Can you work these out from the model? Positions are in its coordinate system, mm. Face numbers are marked on the shaded views. A direction names the side the tool comes from. Coordinates: 2 decimals unless noted, no trailing zeros. Order: outer loops, then holes, each group sorted by start corner. A loop starts at its lowest first (then second) coordinate and runs counter-clockwise, first axis right, second up. Notation, with made-up numbers: M -23.75,89.25 L 1.25,89.25 A28 ccw 1.25,124.25 Z; hole C 47.25,-7.5 d4. An arc over 180 degrees is marked long. Answer as CSV lines item,"result". Start each with the question number.
1. If we section it at A-A (y = -4): List the corners of the cut face in (x, z) for me, plus the area to 3 significant figures.
2. On a 3-axis mill with a long thin cutter (end or side, diameter ignored), from which of +Z, -Z, +X, -X, +Y, -Y can I reach the whole of each face in a straight line? I mean the marked faces 1, 2, 3 and 4. Say none if no direction works.
3. If we section it at B-B (x = 5.75): List the corners of the cut face in (y, z) for me, plus the area to 3 significant figures.
4. If we section it at C-C (z = -8.5): List the corners of the cut face in (x, y) for me, plus the area to 3 significant figures.
5. If we section it at D-D (x = 2.7): List the corners of the cut face in (y, z) for me, plus the area to 3 significant figures.
6. If we mould it in two halves opening along Y, with no side actions, what happens to the marked faces 5, 6, 7 and 8? For each: released by +Y, released by -Y, zero draft, split by the parting line, or undercut.
7. Will these pins go through, and if not, where does the flat tip stop? pin 1 (1.5 mm diameter, centred on x = 4, y = -10.5, fed in from -Z); pin 2 (1.6 mm diameter, centred on y = -3, z = -5, fed in from -X); pin 3 (3.5 mm diameter, centred on x = 4.5, z = -6.5, fed in from -Y).
8. I need wall thicknesses on line 1 along Z through (x, y) = (3.5, -3.25); line 2 along X through (y, z) = (-3.95, -6); line 3 along Y through (x, z) = (6.75, -9). Which ranges of each line are inside material? Lowest first, please. Write a range as from..to.
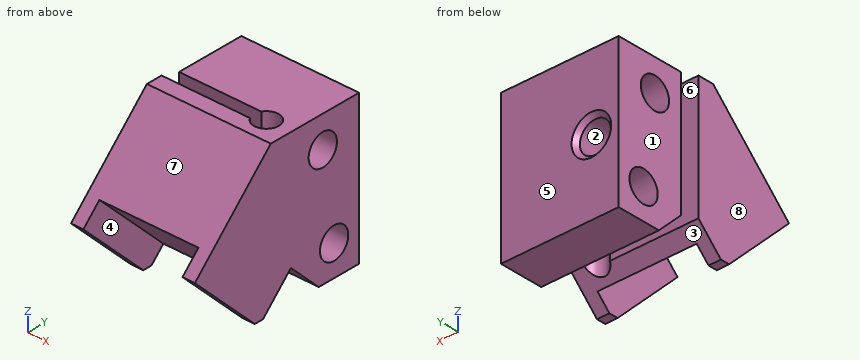
```python
from build123d import *

# Parameters (mm, degrees)
EXTRUDE_1_DEPTH             = 10
SKETCH_2_W                  = 8
SKETCH_2_H                  = 15.737964923
CUT_EXTRUDE_1_DEPTH         = 2
CUT_EXTRUDE_2_DEPTH         = 13
HOLE_WIZARD_M31_D           = 2.5
HOLE_WIZARD_M31_CSINK_D     = 3.3
HOLE_WIZARD_M31_CSINK_ANGLE = 90
HOLE_WIZARD_M32_D           = 2.5
HOLE_WIZARD_M32_DEPTH       = 5.5
HOLE_WIZARD_M32_CSINK_D     = 3.2
HOLE_WIZARD_M32_CSINK_ANGLE = 90
CUT_EXTRUDE_START           = -8
SKETCH_9_W                  = 15.368263211
SKETCH_9_H                  = 5.398005259
CUT_EXTRUDE_3_DEPTH         = 4


with BuildPart() as part:
    # Эскиз1 → Бобышка-Вытянуть1 (new body)
    with BuildSketch(Plane(origin=(0, 0, 0), x_dir=(0, 0, -1), z_dir=(1, 0, 0))):
        Polygon((0, 0), (12, 0), (12, -9.213203436), (6.707106781, -14.506096654), (0, -7.798989873), align=None)
    extrude(amount=EXTRUDE_1_DEPTH)

    # Эскиз2 → Вырез-Вытянуть1 (cut)
    with BuildSketch(Plane(origin=(0, -10.606601718, -10.606601718), x_dir=(-1, 0, 0), z_dir=(0, -0.707106781, -0.707106781))):
        with Locations((-5, -0.262497876)):
            Rectangle(SKETCH_2_W, SKETCH_2_H)
    extrude(amount=-CUT_EXTRUDE_1_DEPTH, mode=Mode.SUBTRACT)

    # Эскиз3 → Вырез-Вытянуть2 (cut, through all)
    with BuildSketch(Plane.XY):
        with BuildLine():
            Line((0.5, -5.5), (0.5, 0))
            Line((0.5, 0), (0, 0))
            Line((0, 0), (0, -6.5))
            Line((0, -6.5), (7.133974596, -6.5))
            ThreePointArc((7.133974596, -6.5), (9, -6), (7.133974596, -5.5))
            Line((7.133974596, -5.5), (0.5, -5.5))
        make_face()
    extrude(amount=-CUT_EXTRUDE_2_DEPTH, mode=Mode.SUBTRACT)

    # Отверстие обработанное метчиком M31 (through all)
    with Locations(Plane.ZY):
        with Locations((-9.535533906, -2.202438662), (-2.535533906, -3.202438662)):
            CounterSinkHole(HOLE_WIZARD_M31_D / 2, HOLE_WIZARD_M31_CSINK_D / 2, counter_sink_angle=HOLE_WIZARD_M31_CSINK_ANGLE)

    # Отверстие обработанное метчиком M32
    with Locations(Plane(origin=(0, 0, 0), x_dir=(-1, 0, 0), z_dir=(0, 1, 0))):
        with Locations((-2.7, -6)):
            CounterSinkHole(HOLE_WIZARD_M32_D / 2, HOLE_WIZARD_M32_CSINK_D / 2, depth=HOLE_WIZARD_M32_DEPTH, counter_sink_angle=HOLE_WIZARD_M32_CSINK_ANGLE)

    # Эскиз9 → Вырез-Вытянуть3 (cut)
    with BuildSketch(Plane(origin=(0, -3.899494937, 3.899494937), x_dir=(1, 0, 0), z_dir=(0, -0.707106781, 0.707106781)).offset(CUT_EXTRUDE_START)):
        with Locations((3.917078905, -13.69900263)):
            Rectangle(SKETCH_9_W, SKETCH_9_H)
    extrude(amount=-CUT_EXTRUDE_3_DEPTH, mode=Mode.SUBTRACT)


solid = part.part
```
Solved:
1,outline,"M 0.5,-11.56 L 10,-11.56 L 10,-3.5 L 0.5,-3.5 Z; M 0.5,-1.57 L 10,-1.57 L 10,0 L 0.5,0 Z; hole C 2.7,-6 d2.5"
1,area,"86.6 mm²"
2,face 1,"+Z, -Z, -X, +Y"
2,face 2,"+Y"
2,face 3,"-Z, +X, -X"
2,face 4,"-Z, -Y"
3,outline,"M -13.09,-5.29 L -7.44,-10.95 L -6.5,-10.01 L -6.5,0 L -7.8,0 Z; M -5.5,-10.06 L -3.56,-12 L 0,-12 L 0,0 L -5.5,0 Z; hole C -3.2,-2.54 d2.5; hole C -2.2,-9.54 d2.5"
3,area,"96.0 mm²"
4,outline,"M 0,-12.71 L 1,-12.71 L 1,-9.88 L 9,-9.88 L 9,-12.71 L 10,-12.71 L 10,-2.9 L 0.5,-2.9 L 0.5,-5.5 L 7.13,-5.5 A1 cw long 7.13,-6.5 L 0,-6.5 Z; M 0.5,-1.5 L 10,-1.5 L 10,0 L 0.5,0 Z"
4,area,"78.3 mm²"
5,outline,"M -13.09,-5.29 L -7.44,-10.95 L -6.5,-10.01 L -6.5,0 L -7.8,0 Z; M -5.5,-10.06 L -3.56,-12 L 0,-12 L 0,-7.6 L -0.35,-7.25 L -5.5,-7.25 Z; M -5.5,-4.75 L -0.35,-4.75 L 0,-4.4 L 0,0 L -5.5,0 Z; hole C -3.2,-2.54 d2.5; hole C -2.2,-9.54 d2.5"
5,area,"82.2 mm²"
6,face 5,"released by +Y"
6,face 6,"undercut"
6,face 7,"released by -Y"
6,face 8,"zero draft"
7,pin 1,"z = -8.63"
7,pin 2,"x = 0.5"
7,pin 3,"y = -13.09"
8,line 1,"-12..-10.22, -8.85..-6.96, -5.04..-3.78, -1.29..0"
8,line 2,"0.5..1.45, 3.95..10"
8,line 3,"-9.38..-6.5, -5.5..-3.33, -1.07..0"
